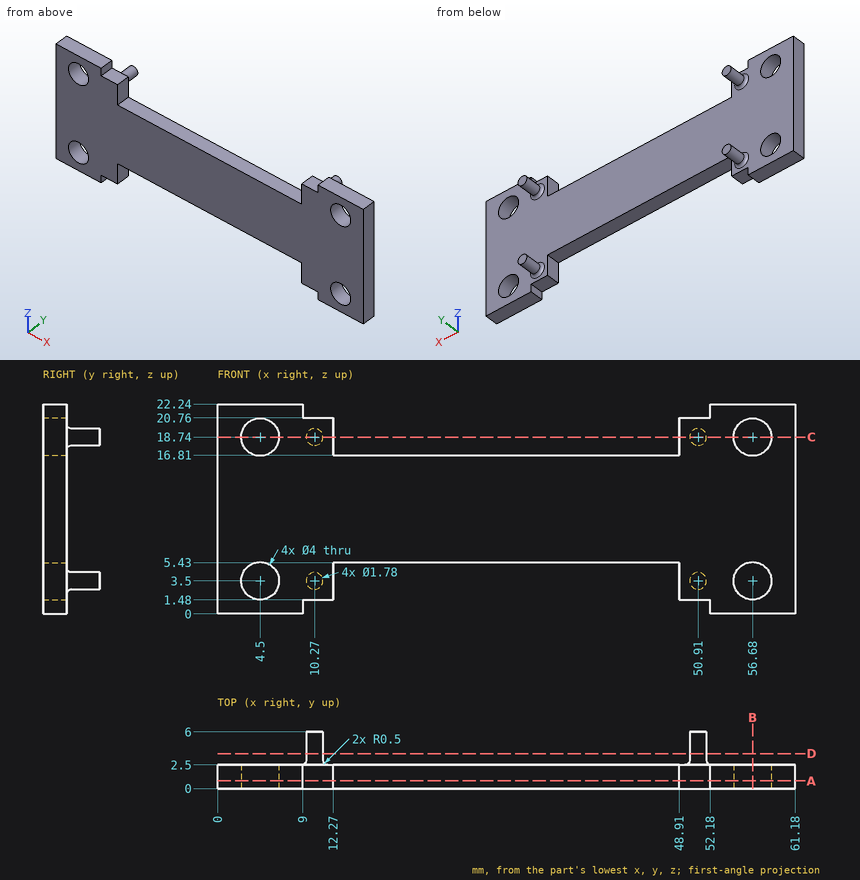
Geometry: see drawing. Coordinates: mm, zero at the bounding-box minimum. Round coordinates to 2 decimals unless told otherwise and drop trailing zeros. Write each loop counter-clockwise with the first axis right and the second up, starting at its lowest first coordinate (ties: lowest second). Pieces come first, ordered by that corner, then holes.
1) Ray query, L1, parallel to X at y = 0.65, z = 3.5; L2, parallel to Y at x = 42.5, z = 16; L3, parallel to Z at x = 22, y = 2.1. Return the intervals inside material, ascending.
2) Cut plane A-A (y = 0.8). Return the cut outline in (x, z).
3) Cut plane B-B (x = 56.68). Return the cut outline in (y, z).
4) Contact query for flat-ended pins moving along their axis: P1, Ø3, axis at x = 4.5, z = 3.5, coming from the +Y side (3 decimals); P2, Ø0.8, axis at x = 51, y = 1.5, coming from the +Z side; P3, Ø4, axis at x = 39, z = 12.5, coming from the -Y side; P4, Ø0.8, axis at x = 10.5, y = 1.5, coming from the -Z side. Output: stop coordinate, or through.
5) Cut plane D-D (y = 3.7). Return the cut outline in (x, z).
6) Cut plane C-C (z = 18.74). Return the cut outline in (x, y), then the cut area to 3 significant figures.
Geometry says:
1. L1: x = 0 to 2.5, 6.5 to 12.27, 48.91 to 54.68, 58.68 to 61.18
1. L2: y = 0 to 2.5
1. L3: z = 5.43 to 16.81
2. outline: (0, 0) - (9, 0) - (9, 1.48) - (12.27, 1.48) - (12.27, 5.43) - (48.91, 5.43) - (48.91, 1.48) - (52.18, 1.48) - (52.18, 0) - (61.18, 0) - (61.18, 22.24) - (52.18, 22.24) - (52.18, 20.76) - (48.91, 20.76) - (48.91, 16.81) - (12.27, 16.81) - (12.27, 20.76) - (9, 20.76) - (9, 22.24) - (0, 22.24) - close; hole circle Ø4 at (4.5, 3.5); hole circle Ø4 at (4.5, 18.74); hole circle Ø4 at (56.68, 3.5); hole circle Ø4 at (56.68, 18.74)
3. outline: (0, 0) - (2.5, 0) - (2.5, 1.5) - (0, 1.5) - close; (0, 5.5) - (2.5, 5.5) - (2.5, 16.74) - (0, 16.74) - close; (0, 20.74) - (2.5, 20.74) - (2.5, 22.24) - (0, 22.24) - close
4. P1: passes through
4. P2: stops at z = 20.76
4. P3: stops at y = 0
4. P4: stops at z = 1.48
5. outline: circle Ø1.78 at (10.27, 3.5); circle Ø1.78 at (10.27, 18.74); circle Ø1.78 at (50.91, 3.5); circle Ø1.78 at (50.91, 18.74)
6. outline: (0, 0) - (2.5, 0) - (2.5, 2.5) - (0, 2.5) - close; (6.5, 0) - (12.27, 0) - (12.27, 2.5) - (11.66, 2.5) arc R0.5 cw to (11.16, 3) - (11.16, 6) - (9.38, 6) - (9.38, 3) arc R0.5 cw to (8.88, 2.5) - (6.5, 2.5) - close; (48.91, 0) - (54.68, 0) - (54.68, 2.5) - (52.3, 2.5) arc R0.5 cw to (51.8, 3) - (51.8, 6) - (50.02, 6) - (50.02, 3) arc R0.5 cw to (49.52, 2.5) - (48.91, 2.5) - close; (58.68, 0) - (61.18, 0) - (61.18, 2.5) - (58.68, 2.5) - close
6. area: 54.0 mm2
